Check sheet for the modelled part. Datum: model origin and axes. Units: mm. A direction names the side the tool comes from. Give positions to 0.01 mm unless a question says otherwise; leave off trailing zeros. Order: outer loops, then holes, each group sorted by start corner. A loop starts at its lowest first (then second) coordinate and runs counter-clockwise, first axis right, second up.
```python
from build123d import *

# Parameters (mm, degrees)
SKETCH1_R           = 42.5
BOSS_EXTRUDE1_DEPTH = 97.5
SKETCH2_R           = 62.5
SKETCH2_R_2         = 42.5
BOSS_EXTRUDE2_DEPTH = 5
SKETCH3_R           = 62.5
SKETCH3_R_2         = 42.5
BOSS_EXTRUDE3_DEPTH = 5
SKETCH4_R           = 90
BOSS_EXTRUDE4_DEPTH = 200
SKETCH6_R           = 12.5
BOSS_EXTRUDE5_DEPTH = 20
CHAMFER1_SIZE       = 7.5
CHAMFER2_SIZE       = 2.5


with BuildPart() as part:
    # Sketch1 → Boss-Extrude1 (new body, symmetric)
    with BuildSketch(Plane.XY):
        with BuildLine():
            Line((100, 100), (100, -100))
            Line((100, -100), (0, -100))
            ThreePointArc((0, -100), (-100, 0), (0, 100))
            Line((0, 100), (100, 100))
        make_face()
        Circle(SKETCH1_R, mode=Mode.SUBTRACT)
    extrude(amount=BOSS_EXTRUDE1_DEPTH, both=True)

    # Sketch2 → Boss-Extrude2 (add)
    with BuildSketch(Plane(origin=(0, 0, -97.5), x_dir=(-1, 0, 0), z_dir=(0, 0, -1))):
        Circle(SKETCH2_R)
        Circle(SKETCH2_R_2, mode=Mode.SUBTRACT)
    extrude(amount=BOSS_EXTRUDE2_DEPTH)

    # Sketch3 → Boss-Extrude3 (add)
    with BuildSketch(Plane.XY.offset(97.5)):
        Circle(SKETCH3_R)
        Circle(SKETCH3_R_2, mode=Mode.SUBTRACT)
    extrude(amount=BOSS_EXTRUDE3_DEPTH)

    # Sketch4 → Boss-Extrude4 (add)
    with BuildSketch(Plane(origin=(100, 0, 0), x_dir=(0, 0, -1), z_dir=(1, 0, 0))):
        Circle(SKETCH4_R)
    extrude(amount=BOSS_EXTRUDE4_DEPTH)

    # Sketch6 → Boss-Extrude5 (add, symmetric)
    with BuildSketch(Plane(origin=(0, 0, 0), x_dir=(1, 0, 0), z_dir=(0, 1, 0))):
        with BuildLine():
            Line((300, -80), (335, -80))
            ThreePointArc((335, -80), (360, -55), (335, -30))
            Line((335, -30), (300, -30))
            Line((300, -30), (300, -80))
        make_face()
        with Locations((335, -55)):
            Circle(SKETCH6_R, mode=Mode.SUBTRACT)
        with BuildLine():
            Line((300, 80), (335, 80))
            ThreePointArc((335, 80), (360, 55), (335, 30))
            Line((335, 30), (300, 30))
            Line((300, 30), (300, 80))
        make_face()
        with Locations((335, 55)):
            Circle(SKETCH6_R, mode=Mode.SUBTRACT)
    extrude(amount=BOSS_EXTRUDE5_DEPTH, both=True)

    # Chamfer1
    chamfer1_edges = [part.edges().sort_by_distance(p)[0] for p in [
        (300, 0, 90),
    ]]
    chamfer(chamfer1_edges, length=CHAMFER1_SIZE)

    # Chamfer2
    chamfer2_edges = [part.edges().sort_by_distance(p)[0] for p in [
        (322.5, -20, 55),
        (322.5, 20, 55),
        (322.5, -20, -55),
        (322.5, 20, -55),
    ]]
    chamfer(chamfer2_edges, length=CHAMFER2_SIZE)


solid = part.part
```
Q1. Go/stop test with flat-tipped pins: P1, Ø1.5, axis at y = 36.5, z = -71.5, coming from the +X side; P2, Ø15, axis at x = 342.5, z = -63, coming from the -Y side; P3, Ø17.5, axis at x = 315, y = -2, coming from the +Z side; P4, Ø22.5, axis at x = 335, z = 55, coming from the -Y side. Record where each tip stops, or that it passes through.
Q2. Draft check along Z on faces 4 (the flat face through (51, -100, 1)), 5 (the flat face through (318, 0, -30)), 6 (the flat face through (317, 0, 80)), 7 (the flat face through (-41, -13, -102.5)). Enter one of: pulls with the +Z half, pulls with the -Z half, needs draft (parallel to the pull), parting line crosses it, or undercut.
Q3. Sectioned sample at A-A, the plane z = 0. Record the cut outline in (x, y), plus the area to 3 significant figures.
Q4. Sectioned sample at B-B, the plane x = 9.5. Record the cut outline in (y, z).
Q5. Tool access check on faces 1 (the flat face through (316, -20, 55)), 2 (the flat face through (317, 20, -55)), 3 (the flat face through (46, -43, 97.5)). Record the directions out of +Z, -Z, +X, -X, +Y, -Y that give a thin tool (end or side, any length) a straight path to the whole face; none if there is none.
Q6. Material ranges on line 1 (Z direction, x = 335, y = 10); line 2 (X direction, y = -0.5, z = -55); line 3 (Y direction, x = 0, z = 99), recorded low to high.
Q7. Sectioned sample at D-D, the plane x = -50.5. Record the cut outline in (y, z).
Q8. Sectioned sample at C-C, the plane z = 55. Count the separate pieces of the cut face and the enclosed holes in it, plus the area to 3 significant figures.
Filled in:
1. P1: stops at x = 300
1. P2: stops at y = -20
1. P3: stops at z = 80
1. P4: passes through
2. face 4: needs draft
2. face 5: undercut
2. face 6: pulls with the +Z half
2. face 7: pulls with the -Z half
3. outline: (0, -100) - (100, -100) - (100, -90) - (292.5, -90) - (300, -82.5) - (300, 82.5) - (292.5, 90) - (100, 90) - (100, 100) - (0, 100) arc R100 ccw to start; hole circle Ø85 at (0, 0)
3. area: 66,000 mm2
4. outline: (-100, -97.5) - (-61.77, -97.5) - (-61.77, -102.5) - (-41.42, -102.5) - (-41.42, 102.5) - (-61.77, 102.5) - (-61.77, 97.5) - (-100, 97.5) - close; (41.42, -102.5) - (61.77, -102.5) - (61.77, -97.5) - (100, -97.5) - (100, 97.5) - (61.77, 97.5) - (61.77, 102.5) - (41.42, 102.5) - close
5. face 1: +Z, -Z, +X, -Y
5. face 2: +Z, -Z, +X, +Y
5. face 3: +Z
6. line 1: z = -80 to -67.5, -42.5 to -30, 30 to 42.5, 67.5 to 80
6. line 2: x = -100 to -42.5, 42.5 to 322.5, 347.5 to 360
6. line 3: y = -62.5 to -42.5, 42.5 to 62.5
7. outline: (-86.31, -97.5) - (-36.82, -97.5) - (-36.82, -102.5) - (36.82, -102.5) - (36.82, -97.5) - (86.31, -97.5) - (86.31, 97.5) - (36.82, 97.5) - (36.82, 102.5) - (-36.82, 102.5) - (-36.82, 97.5) - (-86.31, 97.5) - close
8. separate pieces: 2
8. enclosed holes: 1
8. area: 59,800 mm2
